from build123d import *

# Parameters (mm, degrees)
SKETCH_1_W      = 30
SKETCH_1_H      = 15
EXTRUDE_1_DEPTH = 2
SKETCH_2_W      = 10
SKETCH_2_H      = 3
EXTRUDE_2_DEPTH = 20
EXTRUDE_3_DEPTH = 10
FILLET_2_R      = 3
FILLET_3_R      = 3
FILLET_4_R      = 3
SKETCH_5_W      = 10
SKETCH_5_H      = 1.301428863
EXTRUDE_4_DEPTH = 3
FILLET_5_R      = 3
FILLET_6_R      = 1


with BuildPart() as part:
    # Эскиз1 → Бобышка-Вытянуть1 (new body)
    with BuildSketch(Plane(origin=(0, 0, 0), x_dir=(1, 0, 0), z_dir=(0, 1, 0))):
        Rectangle(SKETCH_1_W, SKETCH_1_H)
    extrude(amount=EXTRUDE_1_DEPTH)

    # Эскиз2 → Бобышка-Вытянуть2 (add)
    with BuildSketch(Plane(origin=(0, 2, 0), x_dir=(1, 0, 0), z_dir=(0, 1, 0))):
        with Locations((0, 6)):
            Rectangle(SKETCH_2_W, SKETCH_2_H)
    extrude(amount=EXTRUDE_2_DEPTH)

    # Эскиз3 → Бобышка-Вытянуть3 (add)
    with BuildSketch(Plane.ZY.offset(5)):
        Polygon((-4.5, 22), (-1.5, 17), (-4.5, 17), align=None)
    extrude(amount=-EXTRUDE_3_DEPTH)

    # Скругление2
    fillet_2_edges = [part.edges().sort_by_distance(p)[0] for p in [
        (0, 22, -4.5),
    ]]
    fillet(fillet_2_edges, radius=FILLET_2_R)

    # Скругление3
    fillet_3_edges = [part.edges().sort_by_distance(p)[0] for p in [
        (0, 2, -4.5),
    ]]
    fillet(fillet_3_edges, radius=FILLET_3_R)

    # Скругление4
    fillet_4_edges = [part.edges().sort_by_distance(p)[0] for p in [
        (-5, 2, -4.5),
        (5, 2, -4.5),
    ]]
    fillet(fillet_4_edges, radius=FILLET_4_R)

    # Эскиз5 → Бобышка-Вытянуть4 (add)
    with BuildSketch(Plane(origin=(0, 22, 0), x_dir=(1, 0, 0), z_dir=(0, 1, 0))):
        with Locations((0, 6.849285569)):
            Rectangle(SKETCH_5_W, SKETCH_5_H)
    extrude(amount=EXTRUDE_4_DEPTH)

    # Скругление5
    fillet_5_edges = [part.edges().sort_by_distance(p)[0] for p in [
        (0, 22, -6.198571137),
    ]]
    fillet(fillet_5_edges, radius=FILLET_5_R)

    # Скругление6
    fillet_6_edges = [part.edges().sort_by_distance(p)[0] for p in [
        (0, 25, -6.198571137),
    ]]
    fillet(fillet_6_edges, radius=FILLET_6_R)


solid = part.part
Can you work these out from the model? Positions are in its coordinate system, mm. A direction names the side the tool comes from. Give positions to 0.01 mm unless a question says otherwise; leave off trailing zeros. Write each loop counter-clockwise with the first axis right and the second up, starting at its lowest first coordinate (ties: lowest second). Pieces come first, ordered by that corner, then holes. Notation, with made-up numbers: M -22,66.25 L -3,66.25 A18 cw -3,85.25 Z; hole C -5.75,59.5 d9. An arc over 180 degrees is marked long. Answer in a Markdown table with one row per item. Add a question column.
Item 1: For pin 1 Ø3 at (x, z) = (0.5, 1) entering from +Y; pin 2 Ø3 at (y, z) = (14.5, -4.5) entering from -X; pin 3 Ø3 at (x, y) = (0.5, 13.5) entering from +Z, each with a flat end and sliding along its axis, tell me the tip position at first contact or that it passes through.
Item 2: Imagine slicing it at B-B, the plane z = 2.75. Write out the boundary of the cut face in (x, y).
Item 3: Imagine slicing it at A-A, the plane z = -3. Write out the boundary of the cut face in (x, y).
Item 4: Please list where these lines run through material, in increasing order: L1, parallel to Z at x = -3.75, y = 16; L2, parallel to Y at x = -8.25, z = 2.75; L3, parallel to Y at x = 0.5, z = -3.
Item 5: On a 3-axis mill with a long thin cutter (end or side, diameter ignored), from which of +Z, -Z, +X, -X, +Y, -Y can I reach the whole of each face in a straight line? I mean faces 1 (the flat face through (0, 10, -7.5)), 2 (the cylindrical face through (-6.252, 2.562, -5.125)), 3 (the flat face through (5, 15, -6)), 4 (the flat face through (0, 2, 2)), 5 (the cylindrical face through (0.11, 2.9, -3.64)). Say none if no direction works.
Item 6: Imagine slicing it at D-D, the plane x = 6.25. Write out the boundary of the cut face in (y, z), plus the area to 3 significant figures.
Item 7: We'd pull the mould along Y, two halves only. Please class faces 6 (the flat face through (0, 0, 0)), 7 (the flat face through (-5, 15, -6)), 8 (the flat face through (0, 11, -4.5)), 9 (the cylindrical face through (6.252, 2.562, -5.125)): released by +Y, released by -Y, zero draft, split by the parting line, or undercut.
Item 8: Imagine slicing it at C-C, the plane y = 14.25. Write out the boundary of the cut face in (x, z), plus the area to 3 significant figures.
Evaluation:
| question | item | result |
|---|---|---|
| 1 | pin 1 | stops at y = 2 |
| 1 | pin 2 | stops at x = -5 |
| 1 | pin 3 | stops at z = -4.5 |
| 2 | outline | M -15,0 L 15,0 L 15,2 L -15,2 Z |
| 3 | outline | M -15,0 L 15,0 L 15,2 L 8,2 A3 cw 6.5,2.4 L -6.5,2.4 A3 cw -8,2 L -15,2 Z; M -5,17 L 5,17 L 5,19.5 L -5,19.5 Z |
| 4 | L1 | z = -7.5 to -4.5 |
| 4 | L2 | y = 0 to 2 |
| 4 | L3 | y = 0 to 2.4, 17 to 19.5 |
| 5 | face 1 | -Z, +X, -X, +Y, -Y |
| 5 | face 2 | +Z, -Z, -X, +Y |
| 5 | face 3 | +Z, -Z, +X, +Y |
| 5 | face 4 | +Z, +Y |
| 5 | face 5 | +Z, +X, -X |
| 6 | outline | M 0,-7.5 L 2.56,-7.5 L 2.56,-3.25 A3 cw 2,-1.5 L 2,7.5 L 0,7.5 Z |
| 6 | area | 32.7 mm² |
| 7 | face 6 | released by -Y |
| 7 | face 7 | zero draft |
| 7 | face 8 | undercut |
| 7 | face 9 | released by +Y |
| 8 | outline | M -5,-7.5 L 5,-7.5 L 5,-4.5 L -5,-4.5 Z |
| 8 | area | 30.0 mm² |
